```python
from build123d import *
from build123d.topology import SkipClean

# Parameters (mm, degrees)
BOSS_EXTRUDE1_START         = 15
SKETCH2_R                   = 5
BOSS_EXTRUDE1_DEPTH         = 15
SKETCH3_R                   = 15
CUT_EXTRUDE1_DEPTH          = 100
F_12_0MM_DOWEL_HOLE1_REACH  = 130.087
F_12_0MM_DOWEL_HOLE1_BORE_R = 6


with BuildPart() as part:
    # Sketch1 → Revolve1 (revolve)
    with BuildSketch(Plane(origin=(0, 0, 0), x_dir=(0, 0, -1), z_dir=(1, 0, 0)), mode=Mode.PRIVATE) as revolve1_sk:
        Polygon((85, 0), (85, 50), (70, 50), (70, 25), (0, 25), (0, 0), align=None)
    revolve(revolve1_sk.sketch.rotate(Axis((0, 0, 0), (0, 0, -1)), 90), axis=Axis((0, 0, 0), (0, 0, -1)))

    # Sketch2 → Boss-Extrude1 (add)
    with SkipClean():  # the faces are left unmerged after this step: merging them gives an invalid solid
        with BuildSketch(Plane.XY.offset(BOSS_EXTRUDE1_START)):
            with BuildLine():
                Line((-6.25, 24.206145914), (-53.125, 12.103072957))
                ThreePointArc((-53.125, 12.103072957), (-62.5, 0), (-53.125, -12.103072957))
                Line((-53.125, -12.103072957), (-6.25, -24.206145914))
                ThreePointArc((-6.25, -24.206145914), (0, -25), (6.25, -24.206145914))
                Line((6.25, -24.206145914), (53.125, -12.103072957))
                ThreePointArc((53.125, -12.103072957), (62.5, 0), (53.125, 12.103072957))
                Line((53.125, 12.103072957), (6.25, 24.206145914))
                ThreePointArc((6.25, 24.206145914), (0, 25), (-6.25, 24.206145914))
            make_face()
            with Locations((-50, 0)):
                Circle(SKETCH2_R, mode=Mode.SUBTRACT)
            with Locations((50, 0)):
                Circle(SKETCH2_R, mode=Mode.SUBTRACT)
        extrude(amount=-BOSS_EXTRUDE1_DEPTH)

    # Sketch3 → Cut-Extrude1 (cut)
    with SkipClean():  # the faces are left unmerged after this step: merging them gives an invalid solid
        with BuildSketch(Plane.XY.offset(15)):
            Circle(SKETCH3_R)
        extrude(amount=-CUT_EXTRUDE1_DEPTH, mode=Mode.SUBTRACT)

    # Ø12.0mm Dowel Hole1 bore → Ø12.0mm Dowel Hole1 (cut, up to next)
    with BuildSketch(Plane(origin=(0, 0, -85), x_dir=(-1, 0, 0), z_dir=(0, 0, -1)), mode=Mode.PRIVATE) as f_12_0mm_dowel_hole1_sk1:
        with Locations((-17.5, -30.310889132)):
            Circle(F_12_0MM_DOWEL_HOLE1_BORE_R)
    f_12_0mm_dowel_hole1_tool1 = extrude(f_12_0mm_dowel_hole1_sk1.sketch, amount=-F_12_0MM_DOWEL_HOLE1_REACH, mode=Mode.PRIVATE) & part.part
    # Ø12.0mm Dowel Hole1 bore → Ø12.0mm Dowel Hole1 (cut, up to next)
    with BuildSketch(Plane(origin=(0, 0, -85), x_dir=(-1, 0, 0), z_dir=(0, 0, -1)), mode=Mode.PRIVATE) as f_12_0mm_dowel_hole1_sk2:
        with Locations((-35, 0)):
            Circle(F_12_0MM_DOWEL_HOLE1_BORE_R)
    f_12_0mm_dowel_hole1_tool2 = extrude(f_12_0mm_dowel_hole1_sk2.sketch, amount=-F_12_0MM_DOWEL_HOLE1_REACH, mode=Mode.PRIVATE) & part.part
    # Ø12.0mm Dowel Hole1 bore → Ø12.0mm Dowel Hole1 (cut, up to next)
    with BuildSketch(Plane(origin=(0, 0, -85), x_dir=(-1, 0, 0), z_dir=(0, 0, -1)), mode=Mode.PRIVATE) as f_12_0mm_dowel_hole1_sk3:
        with Locations((-17.5, 30.310889132)):
            Circle(F_12_0MM_DOWEL_HOLE1_BORE_R)
    f_12_0mm_dowel_hole1_tool3 = extrude(f_12_0mm_dowel_hole1_sk3.sketch, amount=-F_12_0MM_DOWEL_HOLE1_REACH, mode=Mode.PRIVATE) & part.part
    # Ø12.0mm Dowel Hole1 bore → Ø12.0mm Dowel Hole1 (cut, up to next)
    with BuildSketch(Plane(origin=(0, 0, -85), x_dir=(-1, 0, 0), z_dir=(0, 0, -1)), mode=Mode.PRIVATE) as f_12_0mm_dowel_hole1_sk4:
        with Locations((17.5, 30.310889132)):
            Circle(F_12_0MM_DOWEL_HOLE1_BORE_R)
    f_12_0mm_dowel_hole1_tool4 = extrude(f_12_0mm_dowel_hole1_sk4.sketch, amount=-F_12_0MM_DOWEL_HOLE1_REACH, mode=Mode.PRIVATE) & part.part
    # Ø12.0mm Dowel Hole1 bore → Ø12.0mm Dowel Hole1 (cut, up to next)
    with BuildSketch(Plane(origin=(0, 0, -85), x_dir=(-1, 0, 0), z_dir=(0, 0, -1)), mode=Mode.PRIVATE) as f_12_0mm_dowel_hole1_sk5:
        with Locations((35, 0)):
            Circle(F_12_0MM_DOWEL_HOLE1_BORE_R)
    f_12_0mm_dowel_hole1_tool5 = extrude(f_12_0mm_dowel_hole1_sk5.sketch, amount=-F_12_0MM_DOWEL_HOLE1_REACH, mode=Mode.PRIVATE) & part.part
    # Ø12.0mm Dowel Hole1 bore → Ø12.0mm Dowel Hole1 (cut, up to next)
    with BuildSketch(Plane(origin=(0, 0, -85), x_dir=(-1, 0, 0), z_dir=(0, 0, -1)), mode=Mode.PRIVATE) as f_12_0mm_dowel_hole1_sk6:
        with Locations((17.5, -30.310889132)):
            Circle(F_12_0MM_DOWEL_HOLE1_BORE_R)
    f_12_0mm_dowel_hole1_tool6 = extrude(f_12_0mm_dowel_hole1_sk6.sketch, amount=-F_12_0MM_DOWEL_HOLE1_REACH, mode=Mode.PRIVATE) & part.part
    add(f_12_0mm_dowel_hole1_tool1.solids().sort_by_distance((17.5, -30.310889, -85))[0], mode=Mode.SUBTRACT)
    add(f_12_0mm_dowel_hole1_tool2.solids().sort_by_distance((35, 0, -85))[0], mode=Mode.SUBTRACT)
    add(f_12_0mm_dowel_hole1_tool3.solids().sort_by_distance((17.5, 30.310889, -85))[0], mode=Mode.SUBTRACT)
    add(f_12_0mm_dowel_hole1_tool4.solids().sort_by_distance((-17.5, 30.310889, -85))[0], mode=Mode.SUBTRACT)
    add(f_12_0mm_dowel_hole1_tool5.solids().sort_by_distance((-35, 0, -85))[0], mode=Mode.SUBTRACT)
    add(f_12_0mm_dowel_hole1_tool6.solids().sort_by_distance((-17.5, -30.310889, -85))[0], mode=Mode.SUBTRACT)


solid = part.part
```
Read the model definition and answer for the solid it produces. Units are mm, in the model's axes. A direction names the side the tool comes from. Round coordinates to 2 decimals unless told otherwise and drop trailing zeros. Loops run counter-clockwise (first coordinate to the right, second up) from the corner with the lowest first, then second, coordinate; pieces in that order, holes last. Notation, with made-up numbers: (22.5, 75.25) -> (50.5, 75.25) arc R30 ccw to (50.5, 101.25) -> close; hole circle Ø2 at (15, 48.5). An arc over 180 degrees is marked (long way). One line per item, written item: value.
1) A cutting plane is placed at C-C (x = 35). Determine the outline of the cut face in (y, z).
Answer list:
outline: (-35.71, -85) -> (-6, -85) -> (-6, -70) -> (-35.71, -70) -> close; (-16.78, 0) -> (16.78, 0) -> (16.78, 15) -> (-16.78, 15) -> close; (6, -85) -> (35.71, -85) -> (35.71, -70) -> (6, -70) -> close
2) Flat-ended cylindrical pins translate along their axes: P1, Ø1, axis at x = 37, y = -21.5, coming from the +Z side; P2, Ø2, axis at y = -4.5, z = -35, coming from the -X side; P3, Ø11, axis at x = 35, y = 0, coming from the -Z side. Find the tip coordinate at first contact, or state that the pin passes through.
Answer list:
P1: stops at z = -70
P2: stops at x = -24.75
P3: stops at z = 0
3) Consider L1, parallel to Y at x = -17.5, z = -74.5; L2, parallel to Z at x = -39.5, y = -4.5; L3, parallel to Y at x = 0, z = -16. Determine where each line is inside the solid, lowest interval first. Write a range as [from, to].
Answer list:
L1: y = [-46.84, -36.31], [-24.31, 24.31], [36.31, 46.84]
L2: z = [-85, -70], [0, 15]
L3: y = [-25, -15], [15, 25]
4) A cutting plane is placed at A-A (z = 8). Determine the outline of the cut face in (x, y) (3 decimals).
Answer list:
outline: (-53.125, -12.103) -> (-6.25, -24.206) arc R25 ccw to (6.25, -24.206) -> (53.125, -12.103) arc R12.5 ccw to (53.125, 12.103) -> (6.25, 24.206) arc R25 ccw to (-6.25, 24.206) -> (-53.125, 12.103) arc R12.5 ccw to start; hole circle Ø10 at (-50, 0); hole circle Ø30 at (0, 0); hole circle Ø10 at (50, 0)
5) For faces 1 (the face through (-29.36, 18.24, 7.6)), 2 (the face through (45, 0, 8)), 3 (the face through (41, 0, -78)), determine the directions among +Z, -Z, +X, -X, +Y, -Y from which every point of the face is accessible in a straight line to the end or side of a thin tool.
Answer list:
face 1: +Z, -X, +Y
face 2: +Z
face 3: -Z
6) A cutting plane is placed at D-D (z = -8). Determine the outline of the cut face in (x, y), and give its area (3 significant figures).
Answer list:
outline: circle Ø50 at (0, 0); hole circle Ø30 at (0, 0)
area: 1,260 mm²
7) A cutting plane is placed at B-B (x = 0). Determine the outline of the cut face in (y, z), and give its area (3 significant figures).
Answer list:
outline: (-50, -85) -> (-15, -85) -> (-15, 15) -> (-25, 15) -> (-25, -70) -> (-50, -70) -> close; (15, -85) -> (50, -85) -> (50, -70) -> (25, -70) -> (25, 15) -> (15, 15) -> close
area: 2,750 mm²
8) The mould has two halves that part along X. Classify faces 4 (the face through (30.02, 18.07, 7.6)), 5 (the face through (47.69, -15.02, -77.4)), 6 (the face through (-20.269, -35.634, -77.605)): pulls with the +X half, pulls with the -X half, needs draft (parallel to the pull), parting line crosses it, or undercut.
Answer list:
face 4: pulls with the +X half
face 5: parting line crosses it
face 6: undercut
